from build123d import *

# Parameters (mm, degrees)
F3_R          = 2
F4_R          = 3
F6_DEPTH      = 15.0010001
F6_DEPTH_BACK = 15.0010001
F7_T1_DEPTH   = 11.5921148274


# Not quite as in the source:
# - a fillet or chamfer that OpenCascade refuses, or shapes differently, is made with other operations: its cross-section is extruded or revolved along the edge and cut away or added
# - a feature of the source that left no trace in its solid (it failed there, or was rolled back) is left out


with BuildPart() as f1:
    # F0 (on Front) → F1 (revolve)
    with BuildSketch(Plane.XZ):
        Polygon((0, -13.9897428453), (0, 0), (-15, 0), (-15, -3), (-10, -3), (-2.61932757, -13.9897428453), align=None)
    revolve(axis=Axis((0, 0, -6.9948714226), (0, 0, 1)))

    # F2: fillet of radius 10 on 1 edges, made by hand

    # F2_s1 → F2_t2 (revolve)
    with BuildSketch(Plane.XZ):
        with BuildLine():
            ThreePointArc((-15, -3), (-10.4835294041, -4.2493813133), (-7.0321290602, -7.4191283024))
            Line((-7.0321290602, -7.4191283024), (-10, -3))
            Line((-10, -3), (-15, -3))
        make_face()
    revolve(axis=Axis((0, 0, -3), (0, 0, 1)))

    # F3
    f3_edges = [f1.edges().sort_by_distance(p)[0] for p in [
        (15, 0, -3),
    ]]
    fillet(f3_edges, radius=F3_R)

    # F4
    f4_edges = [f1.edges().sort_by_distance(p)[0] for p in [
        (2.619328, 0, -13.989743),
    ]]
    fillet(f4_edges, radius=F4_R)

    # F5 (on Right) → F6 (cut, two sides)
    with BuildSketch(Plane.YZ) as f6_sk:
        with BuildLine():
            Line((1.5, -14.6206104997), (1.5, -12.9897428453))
            ThreePointArc((1.5, -12.9897428453), (0, -8.4897428453), (-1.5, -12.9897428453))
            Line((-1.5, -12.9897428453), (-1.5, -14.6206104997))
            Line((-1.5, -14.6206104997), (1.5, -14.6206104997))
        make_face()
    extrude(amount=-F6_DEPTH, mode=Mode.SUBTRACT)
    extrude(f6_sk.sketch, amount=F6_DEPTH_BACK, mode=Mode.SUBTRACT)

    # F7: fillet of radius 3 on 2 edges, made by hand

    # F7_s2 → F7_t1 (cut)
    with BuildSketch(Plane.YZ.offset(-5.7960574137)):
        with BuildLine():
            ThreePointArc((-2.0454545455, -12.4271417817), (-1.6396122323, -13.2474864717), (-1.5, -14.1520205055))
            Line((-1.5, -14.1520205055), (-1.5, -12.9897428453))
            ThreePointArc((-1.5, -12.9897428453), (-1.7949072323, -12.7299462895), (-2.0454545455, -12.4271417817))
        make_face()
        with BuildLine():
            ThreePointArc((2.0454545455, -12.4271417817), (1.6396122323, -13.2474864717), (1.5, -14.1520205055))
            Line((1.5, -14.1520205055), (1.5, -12.9897428453))
            ThreePointArc((1.5, -12.9897428453), (1.7949072323, -12.7299462895), (2.0454545455, -12.4271417817))
        make_face()
    extrude(amount=F7_T1_DEPTH, mode=Mode.SUBTRACT)


solid = f1.part
Design review of the part built by this model. Coordinates are the model's own, in mm. A direction names the side the tool comes from. Give positions to 0.01 mm unless a question says otherwise; leave off trailing zeros. Loops run counter-clockwise (first coordinate to the right, second up) from the corner with the lowest first, then second, coordinate; pieces in that order, holes last. Notation, with made-up numbers: M -14,82 L 36,82 A8 cw 36,96 Z; hole C -18,-36.5 d5. An arc over 180 degrees is marked long. Write item = value, one per line.
Q1. We need section B-B (z = -8). Give the boundary of the cut face in (x, y), plus the area to 3 significant figures.
Output values:
outline = C 0,0 d13.28
area = 139 mm^2
Q2. For faces 4 (the cylindrical face through (-13.856, 5.745, -0.62)), 5 (the cylindrical face through (-0.043, 1.742, -12.972)), list the 3-axis set-ups (+Z, -Z, +X, -X, +Y, -Y) from which the entire face can be reached by the end or side of a thin tool; tool diameter is ignored.
Output values:
face_4 = +Z, -Z
face_5 = +X, -X
Q3. Insertion check: pin 1 (8 mm diameter, centred on x = 7.5, z = -12, fed in from -Y); pin 2 (4 mm diameter, centred on x = 5.5, z = -1.5, fed in from +Y); pin 3 (4 mm diameter, centred on y = 3.5, z = -6.5, fed in from +X). Each pin has a flat end and moves straight along its axis. Give the tip position at first contact, or say it passes through.
Output values:
pin_1 = -3.55
pin_2 = 14.58
pin_3 = 9.5
Q4. To check wall thickness, follow line 1 (Z direction, x = 2.5, y = 0); line 2 (Y direction, x = 1.5, z = -10.75); line 3 (Y direction, x = -3, z = -10). State the ranges of each line that lie inside material, in increasing order. Write a range as [from, to].
Output values:
line_1 = [-8.49, 0]
line_2 = [-4.55, -2.49], [2.49, 4.55]
line_3 = [-4.37, -2.3], [2.3, 4.37]
Q5. Draft analysis for pull direction Z (two halves, no side actions). For faces 1 (the cylindrical face through (0.09, 0.08, -8.49)), 2 (the conical face through (2.92, 2.24, -12.41)), 3 (the flat face through (0, 0, 0)), state which applies: +Z half, -Z half, draft (parallel to the pull), parting line (faces both ways), or undercut.
Output values:
face_1 = undercut
face_2 = -Z half
face_3 = +Z half
Q6. We need section A-A (z = -10.25). Give the boundary of the cut face in (x, y), plus the area to 3 significant figures.
Output values:
outline = M -4.54,-2.39 A5.13 ccw 4.54,-2.39 Z; M -4.54,2.39 L 4.54,2.39 A5.13 ccw Z
area = 35.5 mm^2
